Could you check a few things on this model? Use its own coordinates, in mm. Coordinates: 2 decimals unless noted, no trailing zeros. Loops run counter-clockwise (first coordinate to the right, second up) from the corner with the lowest first, then second, coordinate; pieces in that order, holes last.
1) Imagine slicing it at C-C on x = 43. Please give me the cut outline in (y, z).
2) Imagine slicing it at B-B on y = -46. Please give me the cut outline in (x, z), plus the area to 3 significant figures.
3) Will these pins go through, and if not, where does the flat tip stop? P1, Ø6, axis at y = 25, z = 50.5, coming from the -X side; P2, Ø4, axis at x = -42.5, z = 28, coming from the +Y side; P3, Ø1, axis at x = 4, z = 32.5, coming from the +Y side.
4) If I drill on line 1 along Y through (x, z) = (-43.5, 42); line 2 along X through (y, z) = (26.5, 31); line 3 along Y through (x, z) = (-29.5, 34), over which ranges is the centre line in solid material (lowest first)?
5) Imagine slicing it at A-A on z = 69.5. Please give me the cut outline in (x, y).
```python
from build123d import *

# Parameters (mm, degrees)
BOX013_W     = 121
BOX013_H     = 121
BOX013_DEPTH = 60.5


with BuildPart() as obj1:
    # Box013 → Box013 (new body)
    with BuildSketch(Plane(origin=(-60.5, -60.5, -45.5), x_dir=(1, 0, 0), z_dir=(0, 0, 1))):
        with Locations((60.5, 60.5)):
            Rectangle(BOX013_W, BOX013_H)
    extrude(amount=BOX013_DEPTH)


with BuildPart() as cockpitglassinnercutter:
    # Sphere001 → Sphere001 (revolve)
    with BuildSketch(Plane(origin=(0, 0, 15), x_dir=(1, 0, 0), z_dir=(0, -1, 0))):
        with BuildLine():
            ThreePointArc((0, -59), (59, 0), (0, 59))
            Line((0, 59), (0, -59))
        make_face()
    revolve(axis=Axis((0, 0, 15), (0, 0, 1)))


with BuildPart() as cockpitglass1:
    # Sphere → Sphere (revolve)
    with BuildSketch(Plane(origin=(0, 0, 15), x_dir=(1, 0, 0), z_dir=(0, -1, 0))):
        with BuildLine():
            ThreePointArc((0, -60.5), (60.5, 0), (0, 60.5))
            Line((0, 60.5), (0, -60.5))
        make_face()
    revolve(axis=Axis((0, 0, 15), (0, 0, 1)))

    # Cut038: cut CockpitGlassInnerCutter
    add(cockpitglassinnercutter.part, mode=Mode.SUBTRACT)

    # Cut039: cut obj1
    add(obj1.part, mode=Mode.SUBTRACT)


solid = cockpitglass1.part
```
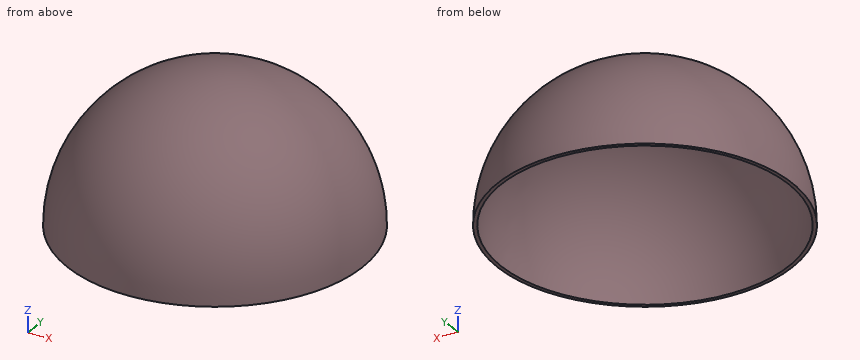
Filled in:
1. outline: (-42.56, 15) - (-40.4, 15) arc R40.4 cw to (40.4, 15) - (42.56, 15) arc R42.56 ccw to start
2. outline: (-39.3, 15) - (-36.95, 15) arc R36.95 cw to (36.95, 15) - (39.3, 15) arc R39.3 ccw to start
2. area: 282 mm2
3. P1: stops at x = -45.02
3. P2: stops at y = 43.11
3. P3: stops at y = 57.93
4. line 1: y = -32.23 to -29.32, 29.32 to 32.23
4. line 2: x = -51.98 to -50.23, 50.23 to 51.98
4. line 3: y = -49.28 to -47.43, 47.43 to 49.28
5. outline: circle Ø52.54 at (0, 0); hole circle Ø45.2 at (0, 0)
